Geometry check sheet. Reference: the model listing, model coordinates, mm. A direction names the side the tool comes from. Give positions to 0.01 mm unless a question says otherwise; leave off trailing zeros. Write each loop counter-clockwise with the first axis right and the second up, starting at its lowest first coordinate (ties: lowest second). Pieces come first, ordered by that corner, then holes. Notation, with made-up numbers: (54, -16.75) - (109, -16.75) arc R11 ccw to (109, -2.75) - close; hole circle Ø4 at (23.25, -20.75). An arc over 180 degrees is marked (long way). Write item = value, one per line. Start each with the question number.
(1) Section check C-C, the plane z = 12. Enter the section's corners in (x, y), plus the area to 3 significant figures.
(2) Access from +Z, -Z, +X, -X, +Y, -Y to the whole of each face (thin tool, end or side, straight path). Record for faces 1 (the cylindrical face through (-5.72, 90.75, 9.14)), 2 (the flat face through (-40, 30, 30)).
(3) Section check B-B, the plane x = -55. Give the number of separate pieces and of enclosed holes in the cut face, plus the area to 3 significant figures.
(4) Depth check by flat-ended pin: pin 1 Ø25 at (x, y) = (-49.5, 44.5) entering from +Z. Enter the tip coordinate at first touch or a pass-through.
(5) Section check D-D, the plane y = 15. Enter the section's corners in (x, z).
(6) Thickness scan on L1, parallel to Z at x = -62, y = 68.5; L2, parallel to Y at x = -54, z = 11; L3, parallel to X at y = -15, z = 30.5. Record the ranges inside material, lowest first.
(7) Draft check along Y on faces 3 (the flat face through (-31, -40.92, 5)), 4 (the flat face through (-15.024, 28, 32)), 5 (the cylindrical face through (-4.829, -32.433, 9.138)). Enter one of: pulls with the +Y half, pulls with the -Y half, needs draft (parallel to the pull), parting line crosses it, or undercut.
```python
from build123d import *
from build123d.topology import SkipClean

# Parameters (mm, degrees)
SKETCH_1_W          = 70
SKETCH_1_H          = 140
EXTRUDE_1_DEPTH     = 10
SKETCH_2_W          = 50
SKETCH_2_H          = 100
EXTRUDE_2_DEPTH     = 20
CHAMFER_2_SIZE      = 20
CHAMFER_3_SIZE      = 20
SKETCH_3_W          = 20
SKETCH_3_H          = 140
EXTRUDE_3_DEPTH     = 25
CUT_EXTRUDE_1_DEPTH = 25
SKETCH_5_R          = 1.5
CUT_EXTRUDE_2_DEPTH = 25


with BuildPart() as part:
    # 草图1 → 凸台-拉伸1 (new body)
    with BuildSketch(Plane.XY):
        with Locations((-30.02391207, 29.079779473)):
            Rectangle(SKETCH_1_W, SKETCH_1_H)
    extrude(amount=EXTRUDE_1_DEPTH)

    # 草图2 → 凸台-拉伸2 (add)
    with BuildSketch(Plane.XY.offset(10)):
        with Locations((-40.02391207, 29.079779473)):
            Rectangle(SKETCH_2_W, SKETCH_2_H)
    extrude(amount=EXTRUDE_2_DEPTH)

    # 倒角2
    chamfer_2_edges = [part.edges().sort_by_distance(p)[0] for p in [
        (-40.02391207, -20.920220527, 10),
    ]]
    chamfer(chamfer_2_edges, length=CHAMFER_2_SIZE - 0.0001)  # a hair under: the kernel refuses the full size

    # 倒角3
    chamfer_3_edges = [part.edges().sort_by_distance(p)[0] for p in [
        (-40.02391207, 79.079779473, 10),
    ]]
    chamfer(chamfer_3_edges, length=CHAMFER_3_SIZE - 0.0001)  # a hair under: the kernel refuses the full size

    # 草图3 → 凸台-拉伸3 (add)
    with BuildSketch(Plane.XY.offset(10)):
        with Locations((-5.02391207, 29.079779473)):
            Rectangle(SKETCH_3_W, SKETCH_3_H)
    extrude(amount=EXTRUDE_3_DEPTH)

    # 草图4 → 切除-拉伸1 (cut)
    with SkipClean():  # the faces are left unmerged after this step: merging them gives an invalid solid
        with BuildSketch(Plane.ZY.offset(15.02391207)):
            Polygon((10, -40.920220527), (42.065793191, -8.854427336), (42.065793191, -55.280550519), align=None)
            Polygon((10, 99.079779473), (42.065793191, 67.013986282), (50.963251555, 103.923082266), align=None)
        extrude(amount=-CUT_EXTRUDE_1_DEPTH, mode=Mode.SUBTRACT)

    # 草图5 → 切除-拉伸2 (cut)
    with SkipClean():  # the faces are left unmerged after this step: merging them gives an invalid solid
        with BuildSketch(Plane(origin=(0, 0, 0), x_dir=(-1, 0, 0), z_dir=(0, 0, -1))):
            with Locations((5.02391207, 92.079779473)):
                Circle(SKETCH_5_R)
            with Locations((55.02391207, 92.079779473)):
                Circle(SKETCH_5_R)
            with Locations((5.02391207, -33.920220527)):
                Circle(SKETCH_5_R)
            with Locations((55.02391207, -33.920220527)):
                Circle(SKETCH_5_R)
        extrude(amount=-CUT_EXTRUDE_2_DEPTH, mode=Mode.SUBTRACT)


solid = part.part
```
Model answer:
q1.outline = (-65.02, -38.92) - (4.98, -38.92) - (4.98, 97.08) - (-65.02, 97.08) - close; hole circle Ø3 at (-55.02, -33.92); hole circle Ø3 at (-55.02, 92.08); hole circle Ø3 at (-5.02, -33.92); hole circle Ø3 at (-5.02, 92.08)
q1.area = 9,490 mm²
q2.face_1 = +Z, -Z
q2.face_2 = +Z, -X, +Y, -Y
q3.separate_pieces = 3
q3.enclosed_holes = 0
q3.area = 3,700 mm²
q4.pin_1 = 30
q5.outline = (-65.02, 0) - (4.98, 0) - (4.98, 35) - (-15.02, 35) - (-15.02, 30) - (-65.02, 30) - close
q6.L1 = 0 to 30
q6.L2 = -39.92 to -35.02, -32.82 to 90.98, 93.18 to 98.08
q6.L3 = -15.02 to 4.98
q7.face_3 = pulls with the -Y half
q7.face_4 = needs draft
q7.face_5 = undercut
